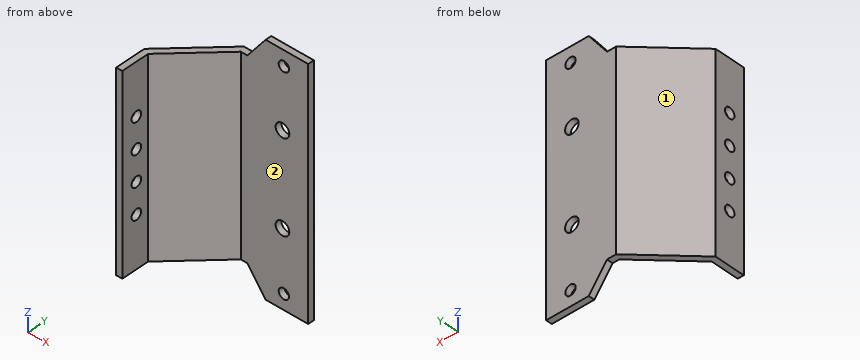
from build123d import *

# Parameters (mm, degrees)
BOSS_EXTRUDE1_DEPTH      = 31.8
M3_CLEARANCE_HOLE1_D     = 3.4
M3_CLEARANCE_HOLE1_DEPTH = 5
M3_CLEARANCE_HOLE1_TIP   = 1.021463052
BOSS_EXTRUDE2_DEPTH      = 2
M3_CLEARANCE_HOLE2_D     = 3.4
M3_CLEARANCE_HOLE2_DEPTH = 5
M3_CLEARANCE_HOLE2_TIP   = 1.021463052
M4_CLEARANCE_HOLE1_D     = 4.5


with BuildPart() as part:
    # Sketch1 → Boss-Extrude1 (new body, symmetric)
    with BuildSketch(Plane.XY):
        Polygon((0, 0), (0, 9.171572875), (15.828427125, 25), (38, 25), (38, 27), (15, 27), (-2, 10), (-2, 0), align=None)
    extrude(amount=BOSS_EXTRUDE1_DEPTH, both=True)

    # M3 Clearance Hole1
    with Locations(Plane(origin=(0, 0, 0), x_dir=(0, 0, -1), z_dir=(1, 0, 0))):
        with Locations((5, 5), (-5, 5), (-15, 5), (15, 5)):
            Hole(M3_CLEARANCE_HOLE1_D / 2, depth=M3_CLEARANCE_HOLE1_DEPTH)
            with Locations((0, 0, -(M3_CLEARANCE_HOLE1_DEPTH + M3_CLEARANCE_HOLE1_TIP / 2))):  # 118° drill point
                Cone(0, M3_CLEARANCE_HOLE1_D / 2, M3_CLEARANCE_HOLE1_TIP, mode=Mode.SUBTRACT)

    # Sketch4 → Boss-Extrude2 (add)
    with BuildSketch(Plane(origin=(0, 27, 0), x_dir=(1, 0, 0), z_dir=(0, 1, 0))):
        Polygon((18, -31.8), (24, -39.8), (38, -39.8), (38, -31.8), align=None)
    boss_extrude2 = extrude(amount=-BOSS_EXTRUDE2_DEPTH)

    # Mirror1: Boss-Extrude2 across plane
    add(boss_extrude2.mirror(Plane.XY))

    # M3 Clearance Hole2
    with Locations(Plane(origin=(0, 27, 0), x_dir=(1, 0, 0), z_dir=(0, 1, 0))):
        with Locations((30, 34.8), (30, -34.8)):
            Hole(M3_CLEARANCE_HOLE2_D / 2, depth=M3_CLEARANCE_HOLE2_DEPTH)
            with Locations((0, 0, -(M3_CLEARANCE_HOLE2_DEPTH + M3_CLEARANCE_HOLE2_TIP / 2))):  # 118° drill point
                Cone(0, M3_CLEARANCE_HOLE2_D / 2, M3_CLEARANCE_HOLE2_TIP, mode=Mode.SUBTRACT)

    # M4 Clearance Hole1 (through all)
    with Locations(Plane(origin=(0, 25, 0), x_dir=(-1, 0, 0), z_dir=(0, -1, 0))):
        with Locations((-29.541515225, 15), (-29.541515225, -15)):
            Hole(M4_CLEARANCE_HOLE1_D / 2)


solid = part.part
Design review of the part built by this model. Coordinates are the model's own, in mm. Face numbers are marked on the shaded views. A direction names the side the tool comes from. Round coordinates to 2 decimals unless told otherwise and drop trailing zeros. Write each loop counter-clockwise with the first axis right and the second up, starting at its lowest first coordinate (ties: lowest second). Pieces come first, ordered by that corner, then holes. Notation, with made-up numbers: (-24.75, 74) - (-10.75, 74) arc R36 ccw to (-10.75, 112) - close; hole circle Ø7 at (28.25, 50.5). An arc over 180 degrees is marked (long way). Use a Markdown table: item, result. Add a question column.
1. Wall thickness on probe 1 along Z at (x, y) = (30, 25.45); probe 2 along Y at (x, z) = (26, -0.5); probe 3 along X at (y, z) = (25.8, 15): over which ranges is each line inside the solid? List them lowest first.
2. We need section B-B (z = 15). State the section outline as (x, y) points.
3. We need section C-C (z = -1). State the section outline as (x, y) points.
4. We need section A-A (z = -34.8). State the section outline as (x, y) points.
5. Clearance check with flat-ended pins moving along their axes: pin 1 (4.5 mm diameter, centred on y = 5, z = 15, fed in from -X); pin 2 (3 mm diameter, centred on y = 5, z = 5, fed in from +X); pin 3 (8 mm diameter, centred on x = 23.5, z = 9.5, fed in from -Y); pin 4 (6 mm diameter, centred on x = 11.5, y = 17.5, fed in from -Z). State where each tip first meets the part, or that it passes through.
6. We need section D-D (y = 2.5). State the section outline as (x, z) points.
7. For the marked faces 1 and 2, list the 3-axis set-ups (+Z, -Z, +X, -X, +Y, -Y) from which the entire face can be reached by the end or side of a thin tool; tool diameter is ignored.
Output:
| question | item | result |
|---|---|---|
| 1 | probe 1 | z = -39.8 to -36.5, -33.1 to -17.2, -12.8 to 12.8, 17.2 to 33.1, 36.5 to 39.8 |
| 1 | probe 2 | y = 25 to 27 |
| 1 | probe 3 | x = 13.8 to 27.29, 31.79 to 38 |
| 2 | outline | (-2, 0) - (0, 0) - (0, 3.3) - (-2, 3.3) - close; (-2, 6.7) - (0, 6.7) - (0, 9.17) - (15.83, 25) - (27.29, 25) - (27.29, 27) - (15, 27) - (-2, 10) - close; (31.79, 25) - (38, 25) - (38, 27) - (31.79, 27) - close |
| 3 | outline | (-2, 0) - (0, 0) - (0, 9.17) - (15.83, 25) - (38, 25) - (38, 27) - (15, 27) - (-2, 10) - close |
| 4 | outline | (20.25, 25) - (28.3, 25) - (28.3, 27) - (20.25, 27) - close; (31.7, 25) - (38, 25) - (38, 27) - (31.7, 27) - close |
| 5 | pin 1 | stops at x = -2 |
| 5 | pin 2 | passes through |
| 5 | pin 3 | stops at y = 25 |
| 5 | pin 4 | stops at z = -31.8 |
| 6 | outline | (-2, -31.8) - (0, -31.8) - (0, 31.8) - (-2, 31.8) - close |
| 7 | face 1 | +Z, -Z, -X, +Y |
| 7 | face 2 | +Z, -Z, +X, -Y |
